Read the model definition and answer for the solid it produces. Units are mm, in the model's axes. A direction names the side the tool comes from. Coordinates: 2 decimals unless noted, no trailing zeros. Write each loop counter-clockwise with the first axis right and the second up, starting at its lowest first coordinate (ties: lowest second). Pieces come first, ordered by that corner, then holes. Notation, with made-up numbers: (84, 46.5) -> (117, 46.5) arc R15 cw to (117, 74.5) -> close; hole circle Ø1 at (54.25, 44.25). An arc over 180 degrees is marked (long way). Answer as a JSON object with one key per item and string values. Group by question number.
(1) For a pull along X with two mould halves and no side action, classify faces 1 (the face through (64.1, 12.68, 31.64)), 2 (the face through (-65, 12, 0)), 3 (the face through (-1, 0, 0)), 4 (the face through (-1, 2, 0)) as +X half, -X half, draft (parallel to the pull), parting line (faces both ways), or undercut.
(2) Find section B-B (z = 25). Give the vertices of the cut face in (x, y), then the cut area to 3 significant figures.
(3) Find section C-C (x = -57.5). Give the vertices of the cut face in (y, z).
(4) Find section A-A (x = -4.5). Give the vertices of the cut face in (y, z).
(5) Find section D-D (z = -20.5). Give the vertices of the cut face in (x, y).
(6) Which of the six approach directions +Z, -Z, +X, -X, +Y, -Y give full straight-line access (tool end or side, diameter ignored) to faces 5 (the face through (64.1, 12.68, -31.64)), 6 (the face through (59, 14, 26))?
(7) Flat-ended cylindrical pins translate along their axes: P1, Ø12, axis at x = -18.5, z = -12, coming from the +Y side; P2, Ø1.6, axis at x = -2.5, z = 31.5, coming from the -Y side; P3, Ø1.5, axis at y = 19, z = 10.5, coming from the +X side; P4, Ø2.5, axis at x = 58.5, z = 25, coming from the +Y side. Find the tip coordinate at first contact, or state that the pin passes through.
(8) Straight lines are drawn through the part: L1, parallel to X at y = 9.4, z = 25; L2, parallel to X at y = 16.5, z = -15; L3, parallel to Z at x = -41.5, y = 24.25. For each, find the intervals that lie inside material, in ascending order.
from build123d import *

# Parameters (mm, degrees)
SKETCH_1_W               = 130
SKETCH_1_H               = 65
EXTRUDE_1_DEPTH          = 25
SKETCH_2_W               = 126
SKETCH_2_H               = 61
CUT_EXTRUDE_1_DEPTH      = 23
SKETCH_3_R               = 2.5
EXTRUDE_2_DEPTH          = 12
SKETCH_5_W               = 8
SKETCH_5_H               = 4
CUT_EXTRUDE_3_DEPTH      = 2
SKETCH_6_W               = 8
SKETCH_6_H               = 3
CUT_EXTRUDE_4_DEPTH      = 2
SKETCH_7_W               = 9
SKETCH_7_H               = 5
CUT_EXTRUDE_5_DEPTH      = 2
SKETCH_8_R               = 1.25
CUT_EXTRUDE_6_DEPTH      = 6
MIRROR_7_COPY_1_SKETCH_R = 2.5
MIRROR_7_COPY_1_DEPTH    = 12
MIRROR_7_COPY_2_SKETCH_R = 1.25
MIRROR_7_COPY_2_DEPTH    = 6
FILLET_1_R               = 1
FILLET_2_R               = 3


with BuildPart() as part:
    # Эскиз1 → Бобышка-Вытянуть1 (new body)
    with BuildSketch(Plane(origin=(0, 0, 0), x_dir=(1, 0, 0), z_dir=(0, 1, 0))):
        Rectangle(SKETCH_1_W, SKETCH_1_H)
    extrude(amount=EXTRUDE_1_DEPTH)

    # Эскиз2 → Вырез-Вытянуть1 (cut)
    with BuildSketch(Plane(origin=(0, 25, 0), x_dir=(1, 0, 0), z_dir=(0, 1, 0))):
        Rectangle(SKETCH_2_W, SKETCH_2_H)
    extrude(amount=-CUT_EXTRUDE_1_DEPTH, mode=Mode.SUBTRACT)

    # Эскиз3 → Бобышка-Вытянуть2 (add)
    with BuildSketch(Plane(origin=(0, 2, 0), x_dir=(1, 0, 0), z_dir=(0, 1, 0))):
        with Locations(Location((-57.5, 25, 0), (0, 0, 90))):
            Circle(SKETCH_3_R)
    extrude_2 = extrude(amount=EXTRUDE_2_DEPTH)

    # Эскиз5 → Вырез-Вытянуть3 (cut)
    with BuildSketch(Plane(origin=(65, 0, 0), x_dir=(0, 0, -1), z_dir=(1, 0, 0))):
        with Locations((0, 20)):
            Rectangle(SKETCH_5_W, SKETCH_5_H)
    cut_extrude_3 = extrude(amount=-CUT_EXTRUDE_3_DEPTH, mode=Mode.SUBTRACT)

    # Зеркальное отражение5: Вырез-Вытянуть3 across plane
    add(cut_extrude_3.mirror(Plane(origin=(0, 0, 0), x_dir=(0, 0, 1), z_dir=(1, 0, 0))), mode=Mode.SUBTRACT)

    # Эскиз6 → Вырез-Вытянуть4 (cut)
    with BuildSketch(Plane.XY.offset(32.5)):
        with Locations((-2.5, 17)):
            Rectangle(SKETCH_6_W, SKETCH_6_H)
    extrude(amount=-CUT_EXTRUDE_4_DEPTH, mode=Mode.SUBTRACT)

    # Эскиз7 → Вырез-Вытянуть5 (cut)
    with BuildSketch(Plane(origin=(65, 0, 0), x_dir=(0, 0, -1), z_dir=(1, 0, 0))):
        with Locations((-12, 18)):
            Rectangle(SKETCH_7_W, SKETCH_7_H)
    extrude(amount=-CUT_EXTRUDE_5_DEPTH, mode=Mode.SUBTRACT)

    # Эскиз8 → Вырез-Вытянуть6 (cut)
    with BuildSketch(Plane(origin=(0, 14, 0), x_dir=(1, 0, 0), z_dir=(0, 1, 0))):
        with Locations(Location((-57.5, 25, 0), (0, 0, 270))):
            Circle(SKETCH_8_R)
    cut_extrude_6 = extrude(amount=-CUT_EXTRUDE_6_DEPTH, mode=Mode.SUBTRACT)

    # Зеркальное отражение6: Бобышка-Вытянуть2, Вырез-Вытянуть6 across plane
    add(extrude_2.mirror(Plane(origin=(0, 0, 0), x_dir=(0, 0, 1), z_dir=(1, 0, 0))))
    add(cut_extrude_6.mirror(Plane(origin=(0, 0, 0), x_dir=(0, 0, 1), z_dir=(1, 0, 0))), mode=Mode.SUBTRACT)

    # Зеркальное отражение7: Бобышка-Вытянуть2, Вырез-Вытянуть6 across plane
    add(extrude_2.mirror(Plane.XY))
    add(cut_extrude_6.mirror(Plane.XY), mode=Mode.SUBTRACT)

    # Зеркальное отражение7 copy 1 sketch → Зеркальное отражение7 copy 1 (add)
    with BuildSketch(Plane(origin=(0, 2, 0), x_dir=(-1, 0, 0), z_dir=(0, 1, 0))):
        with Locations(Location((-57.5, 25, 0), (0, 0, 90))):
            Circle(MIRROR_7_COPY_1_SKETCH_R)
    extrude(amount=MIRROR_7_COPY_1_DEPTH)

    # Зеркальное отражение7 copy 2 sketch → Зеркальное отражение7 copy 2 (cut)
    with BuildSketch(Plane(origin=(0, 14, 0), x_dir=(-1, 0, 0), z_dir=(0, 1, 0))):
        with Locations(Location((-57.5, 25, 0), (0, 0, 270))):
            Circle(MIRROR_7_COPY_2_SKETCH_R)
    extrude(amount=-MIRROR_7_COPY_2_DEPTH, mode=Mode.SUBTRACT)

    # Скругление1
    fillet_1_edges = [part.edges().sort_by_distance(p)[0] for p in [
        (63, 13.5, -30.5),
        (63, 13.5, 30.5),
        (-63, 13.5, 30.5),
        (-63, 13.5, -30.5),
    ]]
    fillet(fillet_1_edges, radius=FILLET_1_R)

    # Скругление2
    fillet_2_edges = [part.edges().sort_by_distance(p)[0] for p in [
        (65, 12.5, 32.5),
        (-65, 12.5, 32.5),
        (-65, 12.5, -32.5),
        (65, 12.5, -32.5),
    ]]
    fillet(fillet_2_edges, radius=FILLET_2_R)


solid = part.part
Results below:
{
 "1": {"face 1": "+X half", "face 2": "-X half", "face 3": "draft", "face 4": "undercut"},
 "2": {"outline": "(-65, 0) -> (65, 0) -> (65, 25) -> (63, 25) -> (63, 2) -> (60, 2) -> (60, 14) -> (58.75, 14) -> (58.75, 8) -> (56.25, 8) -> (56.25, 14) -> (55, 14) -> (55, 2) -> (-55, 2) -> (-55, 14) -> (-56.25, 14) -> (-56.25, 8) -> (-58.75, 8) -> (-58.75, 14) -> (-60, 14) -> (-60, 2) -> (-63, 2) -> (-63, 25) -> (-65, 25) -> close", "area": "442 mm2"},
 "3": {"outline": "(0, -32.5) -> (25, -32.5) -> (25, -30.5) -> (2, -30.5) -> (2, -27.5) -> (14, -27.5) -> (14, -26.25) -> (8, -26.25) -> (8, -23.75) -> (14, -23.75) -> (14, -22.5) -> (2, -22.5) -> (2, 22.5) -> (14, 22.5) -> (14, 23.75) -> (8, 23.75) -> (8, 26.25) -> (14, 26.25) -> (14, 27.5) -> (2, 27.5) -> (2, 30.5) -> (25, 30.5) -> (25, 32.5) -> (0, 32.5) -> close"},
 "4": {"outline": "(0, -32.5) -> (25, -32.5) -> (25, -30.5) -> (2, -30.5) -> (2, 30.5) -> (15.5, 30.5) -> (15.5, 32.5) -> (0, 32.5) -> close; (18.5, 30.5) -> (25, 30.5) -> (25, 32.5) -> (18.5, 32.5) -> close"},
 "5": {"outline": "(-65, 0) -> (65, 0) -> (65, 25) -> (63, 25) -> (63, 2) -> (-63, 2) -> (-63, 25) -> (-65, 25) -> close"},
 "6": {"face 5": "-Z, +X, +Y, -Y", "face 6": "+Y"},
 "7": {"P1": "stops at y = 2", "P2": "stops at y = 0", "P3": "stops at x = -63", "P4": "stops at y = 14"},
 "8": {"L1": "x = -65 to -63, -60 to -58.75, -56.25 to -55, 55 to 56.25, 58.75 to 60, 63 to 65", "L2": "x = -65 to -63, 63 to 65", "L3": "z = -32.5 to -30.5, 30.5 to 32.5"}
}
